Here's how the part is built. I have some questions about the finished solid (model axes, mm). A direction names the side the tool comes from. Give positions to 0.01 mm unless a question says otherwise; leave off trailing zeros. Loops run counter-clockwise (first coordinate to the right, second up) from the corner with the lowest first, then second, coordinate; pieces in that order, holes last. Notation, with made-up numbers: (-40, 57.5) - (-32, 57.5) arc R24 cw to (-32, 91.5) - close; hole circle Ø2 at (65, 15). An arc over 180 degrees is marked (long way). Put each result on its own line as item: value. Start each with the question number.
from build123d import *

# Parameters (mm, degrees)
SKETCH1_R           = 1.5
BOSS_EXTRUDE1_DEPTH = 4


with BuildPart() as part:
    # Sketch1 → Boss-Extrude1 (new body)
    with BuildSketch(Plane.XY):
        with BuildLine():
            Line((-11.169872981, -2.5), (11.169872981, -2.5))
            ThreePointArc((11.169872981, -2.5), (12.151853487, -2.665266452), (13.025641703, -3.142857143))
            ThreePointArc((13.025641703, -3.142857143), (19.5, 0), (13.025641703, 3.142857143))
            ThreePointArc((13.025641703, 3.142857143), (12.151853487, 2.665266452), (11.169872981, 2.5))
            Line((11.169872981, 2.5), (-11.169872981, 2.5))
            ThreePointArc((-11.169872981, 2.5), (-12.151853487, 2.665266452), (-13.025641703, 3.142857143))
            ThreePointArc((-13.025641703, 3.142857143), (-19.5, 0), (-13.025641703, -3.142857143))
            ThreePointArc((-13.025641703, -3.142857143), (-12.151853487, -2.665266452), (-11.169872981, -2.5))
        make_face()
        with Locations((-15.5, 0)):
            Circle(SKETCH1_R, mode=Mode.SUBTRACT)
        with Locations(Location((15.5, 0, 0), (0, 0, 180))):
            Circle(SKETCH1_R, mode=Mode.SUBTRACT)
    extrude(amount=BOSS_EXTRUDE1_DEPTH)


solid = part.part
1) I'm going to push flat-ended pins straight in: P1, Ø3, axis at x = -4.5, y = -3, coming from the +Z side; P2, Ø2, axis at x = 1.5, z = 1.5, coming from the -Y side; P3, Ø2, axis at x = 4, z = 2, coming from the +Y side. Where does each tip first touch, or does it pass through?
2) Suppose I cut it at C-C on z = 0.4. Please give me the cut outline in (x, y).
3) Thinking about a two-plate mould opening in Y: for faces 1 (the cylindrical face through (-17, 0, 2)), 2 (the cylindrical face through (-19.5, 0.1, 2)), 3 (the flat face through (0, 2.5, 2)), which applies, pulls with the +Y half, pulls with the -Y half, needs draft (parallel to the pull), parting line crosses it, or undercut?
4) Which directions (+Z, -Z, +X, -X, +Y, -Y) give clear straight access to the entire face, cutting with the end or side of a thin tool? Please do faces 4 (the cylindrical face through (-12.14, 2.66, 1.97)), 5 (the flat face through (0, -2.5, 2)), 6 (the cylindrical face through (17, 0, 2)).
5) Suppose I cut it at D-D on x = -10. Please give me the cut outline in (y, z).
6) I need wall thicknesses on line 1 (Y direction, x = -3.5, z = 3.8); line 2 (X direction, y = -1, z = 3.7); line 3 (Y direction, x = 13.5, z = 0.65). Which ranges of each line are inside material? Lowest first, please.
7) Suppose I cut it at A-A on x = -15.5. Please give me the cut outline in (y, z).
8) Suppose I cut it at B-B on y = 0. Please give me the cut outline in (x, z), plus the area to 3 significant figures.
Ans:
1. P1: stops at z = 4
1. P2: stops at y = -2.5
1. P3: stops at y = 2.5
2. outline: (-13.03, -3.14) arc R3 cw to (-11.17, -2.5) - (11.17, -2.5) arc R3 cw to (13.03, -3.14) arc R4 ccw (long way) to (13.03, 3.14) arc R3 cw to (11.17, 2.5) - (-11.17, 2.5) arc R3 cw to (-13.03, 3.14) arc R4 ccw (long way) to start; hole circle Ø3 at (-15.5, 0); hole circle Ø3 at (15.5, 0)
3. face 1: undercut
3. face 2: parting line crosses it
3. face 3: pulls with the +Y half
4. face 4: +Z, -Z, +Y
4. face 5: +Z, -Z, -Y
4. face 6: +Z, -Z
5. outline: (-2.5, 0) - (2.5, 0) - (2.5, 4) - (-2.5, 4) - close
6. line 1: y = -2.5 to 2.5
6. line 2: x = -19.37 to -16.62, -14.38 to 14.38, 16.62 to 19.37
6. line 3: y = -3.46 to 3.46
7. outline: (-4, 0) - (-1.5, 0) - (-1.5, 4) - (-4, 4) - close; (1.5, 0) - (4, 0) - (4, 4) - (1.5, 4) - close
8. outline: (-19.5, 0) - (-17, 0) - (-17, 4) - (-19.5, 4) - close; (-14, 0) - (14, 0) - (14, 4) - (-14, 4) - close; (17, 0) - (19.5, 0) - (19.5, 4) - (17, 4) - close
8. area: 132 mm²
